The model under review builds one solid part; all positions refer to its coordinate system, in mm. Coordinates: 2 decimals unless noted, no trailing zeros. Order: outer loops, then holes, each group sorted by start corner. A loop starts at its lowest first (then second) coordinate and runs counter-clockwise, first axis right, second up. Notation, with made-up numbers: M 14,36 L 20,36 A27 cw 20,65 Z; hole C 19,2.25 d8. An arc over 180 degrees is marked long. Answer in a Markdown table with one row per item.
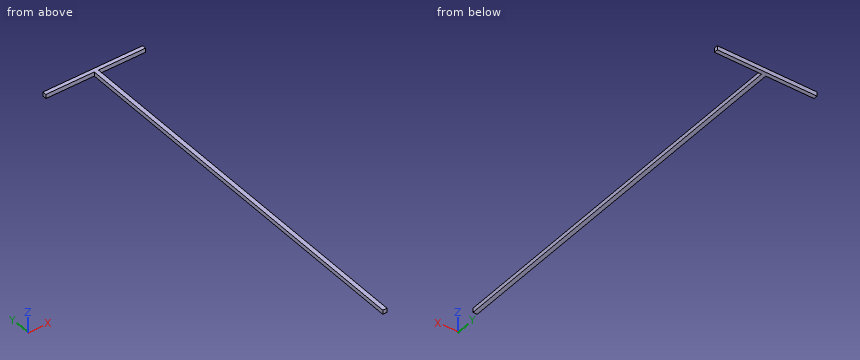
from build123d import *

# Parameters (mm, degrees)
SKETCH_1_W      = 238.070236771
SKETCH_1_H      = 9.336087717
SKETCH_1_W_2    = 10
SKETCH_1_H_2    = 918.957046125
EXTRUDE_1_DEPTH = 10


with BuildPart() as part:
    # Эскиз1 → Бобышка-Вытянуть1 (new body)
    with BuildSketch(Plane.XY):
        with Locations((53.68250437, 36.177339902)):
            Rectangle(SKETCH_1_W, SKETCH_1_H)
        with Locations((55.096797899, -427.96922702)):
            Rectangle(SKETCH_1_W_2, SKETCH_1_H_2)
    extrude(amount=EXTRUDE_1_DEPTH)


solid = part.part
(1) Take a section at A-A (z = 6). Write out the cut boundary in (x, y), then the cut area to 3 significant figures.
Report:
| item | result |
|---|---|
| outline | M -65.35,31.51 L 50.1,31.51 L 50.1,-887.45 L 60.1,-887.45 L 60.1,31.51 L 172.72,31.51 L 172.72,40.85 L -65.35,40.85 Z |
| area | 11,400 mm^2 |
(2) To check wall thickness, follow line 1 (Y direction, x = -3, z = 7.5); line 2 (X direction, y = -769.5, z = 6.25). State the ranges of each line that lie inside material, in increasing order. Write a range as [from, to].
Report:
| item | result |
|---|---|
| line 1 | [31.51, 40.85] |
| line 2 | [50.1, 60.1] |
(3) Insertion check: P1, Ø6, axis at x = 102, z = 1.5, coming from the -Y side; P2, Ø3, axis at y = -432.5, z = 7.5, coming from the -X side; P3, Ø3, axis at y = -336.5, z = 5.5, coming from the +X side. Each pin has a flat end and moves straight along its axis. Give the tip position at first contact, or say it passes through.
Report:
| item | result |
|---|---|
| P1 | y = 31.51 |
| P2 | x = 50.1 |
| P3 | x = 60.1 |
(4) Take a section at C-C (y = -55). Write out the cut boundary in (x, z).
Report:
| item | result |
|---|---|
| outline | M 50.1,0 L 60.1,0 L 60.1,10 L 50.1,10 Z |
(5) Take a section at B-B (x = -20.5). Write out the cut boundary in (y, z), then the cut area to 3 significant figures.
Report:
| item | result |
|---|---|
| outline | M 31.51,0 L 40.85,0 L 40.85,10 L 31.51,10 Z |
| area | 93.4 mm^2 |
